from build123d import *

# Parameters (mm, degrees)
SKETCH1_R                                         = 15.875
SKETCH1_R_2                                       = 5.55625
BOSS_EXTRUDE1_DEPTH                               = 3.175
CSK_FOR_6_FLAT_HEAD_MACHINE_SCREW_100_D           = 3.7973
CSK_FOR_6_FLAT_HEAD_MACHINE_SCREW_100_CSINK_D     = 7.0866
CSK_FOR_6_FLAT_HEAD_MACHINE_SCREW_100_CSINK_ANGLE = 100


with BuildPart() as part:
    # Sketch1 → Boss-Extrude1 (new body)
    with BuildSketch(Plane(origin=(0, 0, 0), x_dir=(1, 0, 0), z_dir=(0, 1, 0))):
        with Locations(Location((0, 0, 0), (0, 0, 270))):
            Circle(SKETCH1_R)
        with Locations(Location((0, 0, 0), (0, 0, 270))):
            Circle(SKETCH1_R_2, mode=Mode.SUBTRACT)
    extrude(amount=BOSS_EXTRUDE1_DEPTH)

    # CSK for #6 Flat Head Machine Screw (100)1 (through all)
    with Locations(Plane(origin=(0, 3.175, 0), x_dir=(1, 0, 0), z_dir=(0, 1, 0))):
        with Locations((0, -10.31875), (0, 10.31875)):
            CounterSinkHole(CSK_FOR_6_FLAT_HEAD_MACHINE_SCREW_100_D / 2, CSK_FOR_6_FLAT_HEAD_MACHINE_SCREW_100_CSINK_D / 2, counter_sink_angle=CSK_FOR_6_FLAT_HEAD_MACHINE_SCREW_100_CSINK_ANGLE)


solid = part.part
Source: CAD feature listing. Evaluate the final solid. Frame: model axes, mm. Round coordinates to 2 decimals unless told otherwise and drop trailing zeros. Loops run counter-clockwise (first coordinate to the right, second up) from the corner with the lowest first, then second, coordinate; pieces in that order, holes last. Notation, with made-up numbers: (27, -14.75) -> (79, -14.75) arc R17 cw to (79, -10.75) -> close; hole circle Ø6 at (40, 25). An arc over 180 degrees is marked (long way). Answer as a JSON object with one key per item and string values. Group by question number.
Q1. Section query A-A (x = 0). Output: boundary loops of the cut face in (y, z) (3 decimals).
Q2. Ray query, line 1 (X direction, y = 2.7, z = -1.5); line 2 (Z direction, x = -1, y = 0.95); line 3 (X direction, y = 2.3, z = 8.5). Return the intervals inside material, ascending. Write a range as from..to.
Q3. Contact query for flat-ended pins moving along their axis: P1, Ø1.5, axis at y = 0.5, z = -1.5, coming from the -X side; P2, Ø9, axis at x = 0, z = 0, coming from the +Y side; P3, Ø12, axis at x = -0.5, z = -10.5, coming from the +Y side (3 decimals); P4, Ø1.5, axis at x = -11.5, y = 0.5, coming from the -Z side. Output: stop coordinate, or through.
Q4. Mould query, pull axis Z, two halves, no side actions, for faces 1 (the cylindrical face through (-15.497, 1.565, -3.441)), 2 (the cylindrical face through (4.685, 1.565, 2.987)), 3 (the flat face through (-7, 3.175, 0)). Classes: pulls with the +Z half, pulls with the -Z half, needs draft (parallel to the pull), parting line crosses it, or undercut.
Q5. Section query D-D (y = 0.95). State how many separate pieces and enclosed holes the cut face has, plus the area to 3 significant figures.
Q6. Section query C-C (x = 4). Output: boundary loops of the cut face in (y, z) (3 decimals), plus the area to 3 significant figures.
Q7. Section query B-B (z = 0). Output: boundary loops of the cut face in (x, y) (3 decimals), plus the area to 3 significant figures.
Completed:
{
 "1": {"outline": "(0, -15.875) -> (3.175, -15.875) -> (3.175, -13.862) -> (1.795, -12.217) -> (0, -12.217) -> close; (0, -8.42) -> (1.795, -8.42) -> (3.175, -6.775) -> (3.175, -5.556) -> (0, -5.556) -> close; (0, 5.556) -> (3.175, 5.556) -> (3.175, 6.775) -> (1.795, 8.42) -> (0, 8.42) -> close; (0, 12.217) -> (1.795, 12.217) -> (3.175, 13.862) -> (3.175, 15.875) -> (0, 15.875) -> close"},
 "2": {"line 1": "-15.8..-5.35, 5.35..15.8", "line 2": "-15.84..-11.93, -8.7..-5.47, 5.47..8.7, 11.93..15.84", "line 3": "-13.41..-1.72, 1.72..13.41"},
 "3": {"P1": "x = -15.86", "P2": "through", "P3": "y = 3.175", "P4": "z = -11.68"},
 "4": {"face 1": "parting line crosses it", "face 2": "undercut", "face 3": "needs draft"},
 "5": {"separate pieces": "1", "enclosed holes": "3", "area": "672 mm²"},
 "6": {"outline": "(0, -15.363) -> (3.175, -15.363) -> (3.175, -3.856) -> (0, -3.856) -> close; (0, 3.856) -> (3.175, 3.856) -> (3.175, 15.363) -> (0, 15.363) -> close", "area": "73.1 mm²"},
 "7": {"outline": "(-15.875, 0) -> (-5.556, 0) -> (-5.556, 3.175) -> (-15.875, 3.175) -> close; (5.556, 0) -> (15.875, 0) -> (15.875, 3.175) -> (5.556, 3.175) -> close", "area": "65.5 mm²"}
}
